Geometry: see drawing. Coordinates: mm, zero at the bounding-box minimum. A direction names the side the tool comes from. Coordinates: 2 decimals unless noted, no trailing zeros. Write each loop counter-clockwise with the first axis right and the second up, starting at its lowest first coordinate (ties: lowest second). Pieces come first, ordered by that corner, then holes.
1) Section query D-D (y = 7). Output: boundary loops of the cut face in (x, z).
2) Pin query (flat end, axial travel): pin 1 Ø5 at (x, z) = (27, 6) entering from +Y; pin 2 Ø1.5 at (x, z) = (51, 14) entering from -Y; pin 3 Ø6 at (x, z) = (43, 3) entering from -Y; pin 4 Ø10 at (x, y) = (33.5, 29) entering from -Z. Return the tip coordinate at first contact, or that it passes through.
3) Section query A-A (y = 30.5). Output: boundary loops of the cut face in (x, z), then the cut area to 4 significant figures.
4) Set-up query: the marked faces 1 and 2. Return all of +Z, -Z, +X, -X, +Y, -Y with unobstructed straight access to the full face (end or side cutting, diameter ignored); none if empty.
5) Draft query along Z for the marked faces 3, 4 and 5. Return one class per face: pulls with the +Z half, pulls with the -Z half, needs draft (parallel to the pull), parting line crosses it, or undercut.
6) Section query C-C (z = 5.25). Output: boundary loops of the cut face in (x, y), then the cut area to 3 significant figures.
7) Line query: L1, parallel to Y at x = 30.5, z = 6.25; L2, parallel to Z at x = 18, y = 11; L3, parallel to Y at x = 30.5, z = 11.5. Output: solid intervals per line, ascending.
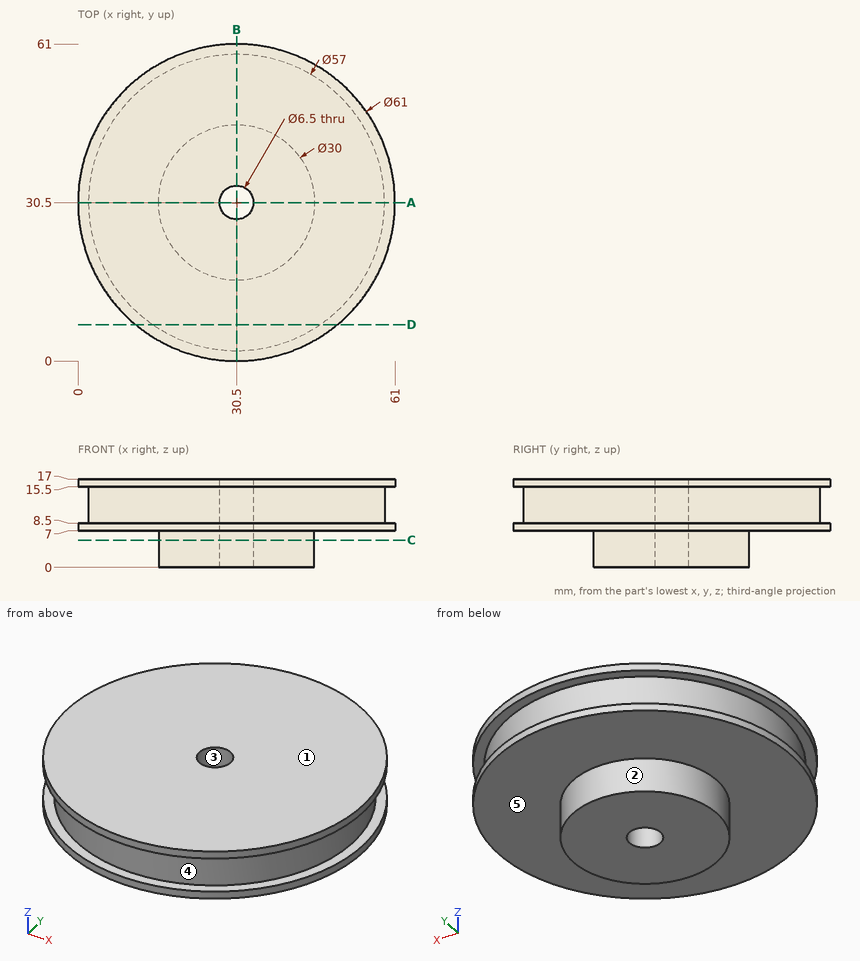
Answer:
1. outline: (11.06, 7) - (49.94, 7) - (49.94, 8.5) - (46.62, 8.5) - (46.62, 15.5) - (49.94, 15.5) - (49.94, 17) - (11.06, 17) - (11.06, 15.5) - (14.38, 15.5) - (14.38, 8.5) - (11.06, 8.5) - close
2. pin 1: stops at y = 60.98
2. pin 2: stops at y = 9.95
2. pin 3: stops at y = 18.89
2. pin 4: stops at z = 0
3. outline: (0, 7) - (15.5, 7) - (15.5, 0) - (27.25, 0) - (27.25, 17) - (0, 17) - (0, 15.5) - (2, 15.5) - (2, 8.5) - (0, 8.5) - close; (33.75, 0) - (45.5, 0) - (45.5, 7) - (61, 7) - (61, 8.5) - (59, 8.5) - (59, 15.5) - (61, 15.5) - (61, 17) - (33.75, 17) - close
3. area: 681.5 mm2
4. face 1: +Z, +X, -X, +Y, -Y
4. face 2: -Z
5. face 3: needs draft
5. face 4: undercut
5. face 5: pulls with the -Z half
6. outline: circle Ø30 at (30.5, 30.5); hole circle Ø6.5 at (30.5, 30.5)
6. area: 674 mm2
7. L1: y = 15.5 to 27.25, 33.75 to 45.5
7. L2: z = 7 to 17
7. L3: y = 2 to 27.25, 33.75 to 59
